```python
from build123d import *

# Parameters (mm, degrees)
PAD_DEPTH    = 12
POCKET_DEPTH = 12.001
FILLET_R     = 0.2
FILLET001_R  = 0.2


with BuildPart() as part:
    # Sketch → Pad (new body)
    with BuildSketch(Plane.XY):
        with BuildLine():
            ThreePointArc((5, 2), (0, 7), (-5, 2))
            Line((-5, 2), (-5, -2))
            ThreePointArc((-5, -2), (0, -7), (5, -2))
            Line((5, -2), (5, 2))
        make_face()
    extrude(amount=-PAD_DEPTH)

    # Sketch001 (on Face6 of Pad) → Pocket (cut, through all)
    with BuildSketch(Plane(origin=(0, 0, -12), x_dir=(1, 0, 0), z_dir=(0, 0, -1))):
        with BuildLine():
            ThreePointArc((4.15, 2.1), (0, 6.25), (-4.15, 2.1))
            Line((-4.15, 2.1), (-4.15, -2.1))
            ThreePointArc((-4.15, -2.1), (0, -6.25), (4.15, -2.1))
            Line((4.15, -2.1), (4.15, 2.1))
        make_face()
    extrude(amount=-POCKET_DEPTH, mode=Mode.SUBTRACT)

    # Fillet
    fillet_edges = [part.edges().sort_by_distance(p)[0] for p in [
        (0, 7, 0),
        (5, 0, 0),
        (-5, 0, 0),
        (0, -7, 0),
        (4.15, 0, 0),
        (0, 6.25, 0),
        (-4.15, 0, 0),
        (0, -6.25, 0),
    ]]
    fillet(fillet_edges, radius=FILLET_R)

    # Fillet001
    fillet001_edges = [part.edges().sort_by_distance(p)[0] for p in [
        (0, 7, -12),
        (5, 0, -12),
        (-5, 0, -12),
        (0, -7, -12),
        (4.15, 0, -12),
        (0, 6.25, -12),
        (-4.15, 0, -12),
        (0, -6.25, -12),
    ]]
    fillet(fillet001_edges, radius=FILLET001_R)


solid = part.part
```
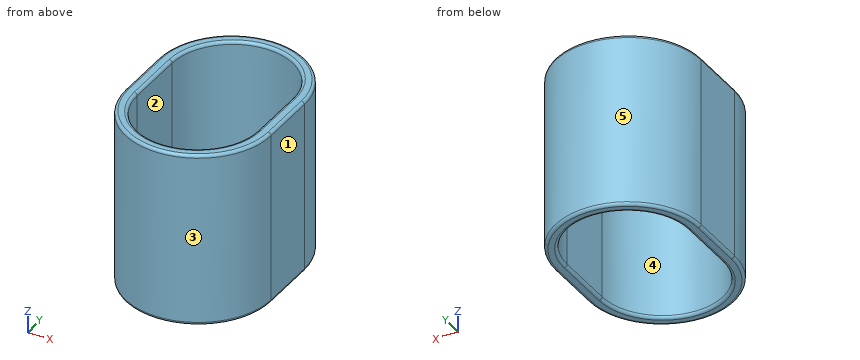
Can you work these out from the model? Positions are in its coordinate system, mm. Face numbers are marked on the shaded views. A direction names the side the tool comes from. Round coordinates to 2 decimals unless told otherwise and drop trailing zeros. Loops run counter-clockwise (first coordinate to the right, second up) from the corner with the lowest first, then second, coordinate; pieces in that order, holes last.
Item 1: Suppose I cut it at B-B, the plane z = -3. Write out the boundary of the cut face in (x, y).
Item 2: If we mould it in two halves opening along Y, with no side actions, what happens to the marked faces 1, 2 and 3? For each: +Y half, -Y half, draft (parallel to the pull), parting line (faces both ways), or undercut.
Item 3: Please list where these lines run through material, in increasing order: L1, parallel to X at y = -0.5, z = -6.5; L2, parallel to X at y = 5.75, z = -7.5; L3, parallel to Y at x = 0.75, z = -1.5.
Item 4: Will these pins go through, and if not, where does the flat tip stop? pin 1 Ø2 at (x, z) = (-3.5, -6) entering from +Y; pin 2 Ø2 at (x, y) = (-3.5, 1) entering from -Z; pin 3 Ø2 at (x, y) = (-0.5, 4.5) entering from +Z; pin 4 Ø2 at (x, z) = (2, -4) entering from +Y.
Item 5: Which directions (+Z, -Z, +X, -X, +Y, -Y) give clear straight access to the entire face, cutting with the end or side of a thin tool? Please do the marked faces 4 and 5.
Item 6: Suppose I cut it at A-A, the plane y = -1.75. Write out the boundary of the cut face in (x, z).
Item 7: Suppose I cut it at C-C, the plane x = 0. Write out the boundary of the cut face in (y, z).
Reported:
1. outline: (-5, -2) arc R5 ccw to (5, -2) - (5, 2) arc R5 ccw to (-5, 2) - close; hole (-4.15, -2.1) arc R4.15 ccw to (4.15, -2.1) - (4.15, 2.1) arc R4.15 ccw to (-4.15, 2.1) - close
2. face 1: draft
2. face 2: undercut
2. face 3: -Y half
3. L1: x = -5 to -4.15, 4.15 to 5
3. L2: x = -3.31 to -1.97, 1.97 to 3.31
3. L3: y = -6.94 to -6.18, 6.18 to 6.94
4. pin 1: stops at y = 6.33
4. pin 2: stops at z = -12
4. pin 3: passes through
4. pin 4: stops at y = 6.9
5. face 4: +Z, -Z
5. face 5: +Z, -Z, +Y
6. outline: (-5, -11.8) arc R0.2 ccw to (-4.8, -12) - (-4.35, -12) arc R0.2 ccw to (-4.15, -11.8) - (-4.15, -0.2) arc R0.2 ccw to (-4.35, 0) - (-4.8, 0) arc R0.2 ccw to (-5, -0.2) - close; (4.15, -11.8) arc R0.2 ccw to (4.35, -12) - (4.8, -12) arc R0.2 ccw to (5, -11.8) - (5, -0.2) arc R0.2 ccw to (4.8, 0) - (4.35, 0) arc R0.2 ccw to (4.15, -0.2) - close
7. outline: (-7, -11.8) arc R0.2 ccw to (-6.8, -12) - (-6.45, -12) arc R0.2 ccw to (-6.25, -11.8) - (-6.25, -0.2) arc R0.2 ccw to (-6.45, 0) - (-6.8, 0) arc R0.2 ccw to (-7, -0.2) - close; (6.25, -11.8) arc R0.2 ccw to (6.45, -12) - (6.8, -12) arc R0.2 ccw to (7, -11.8) - (7, -0.2) arc R0.2 ccw to (6.8, 0) - (6.45, 0) arc R0.2 ccw to (6.25, -0.2) - close
